```python
from build123d import *

# Parameters (mm, degrees)
SKETCH1_R           = 3.2639
BOSS_EXTRUDE1_DEPTH = 4.7752


with BuildPart() as part:
    # Sketch1 → Boss-Extrude1 (new body)
    with BuildSketch(Plane.XY):
        with BuildLine():
            Line((-76.2, 0), (0, 0))
            Line((0, 0), (0, 76.2))
            Line((0, 76.2), (-24.638, 76.2))
            Line((-24.638, 76.2), (-24.638, 27.0256))
            ThreePointArc((-24.638, 27.0256), (-25.337311849, 25.337311849), (-27.0256, 24.638))
            Line((-27.0256, 24.638), (-76.2, 24.638))
            Line((-76.2, 24.638), (-76.2, 0))
        make_face()
        with Locations((-12.7, 38.1)):
            Circle(SKETCH1_R, mode=Mode.SUBTRACT)
        with Locations((-12.7, 63.5)):
            Circle(SKETCH1_R, mode=Mode.SUBTRACT)
        with Locations((-12.7, 12.7)):
            Circle(SKETCH1_R, mode=Mode.SUBTRACT)
        with Locations((-38.1, 12.7)):
            Circle(SKETCH1_R, mode=Mode.SUBTRACT)
        with Locations((-63.5, 12.7)):
            Circle(SKETCH1_R, mode=Mode.SUBTRACT)
    extrude(amount=BOSS_EXTRUDE1_DEPTH)


solid = part.part
```
Design review of the part built by this model. Coordinates are the model's own, in mm. A direction names the side the tool comes from. Coordinates: 2 decimals unless noted, no trailing zeros. Write each loop counter-clockwise with the first axis right and the second up, starting at its lowest first coordinate (ties: lowest second). Pieces come first, ordered by that corner, then holes. Notation, with made-up numbers: M 64,13 L 97,13 A29 ccw 97,41 Z; hole C 35,40.25 d2. An arc over 180 degrees is marked long. Answer as a JSON object with one key per item and string values.
Item 1: Draft analysis for pull direction X (two halves, no side actions). For faces 1 (the flat face through (-30, 22, 4.775)), 2 (the cylindrical face through (-13.125, 41.336, 2.354)), 3 (the cylindrical face through (-25.319, 25.356, 2.354)), state which applies: pulls with the +X half, pulls with the -X half, needs draft (parallel to the pull), parting line crosses it, or undercut.
Outcome:
{"face 1": "needs draft", "face 2": "undercut", "face 3": "pulls with the -X half"}
Item 2: Add section C-C, the plane z = 3.95. Give the boundary of the cut face in (x, y), and give its area (3 significant figures).
Outcome:
{"outline": "M -76.2,0 L 0,0 L 0,76.2 L -24.64,76.2 L -24.64,27.03 A2.39 cw -27.03,24.64 L -76.2,24.64 Z; hole C -63.5,12.7 d6.53; hole C -38.1,12.7 d6.53; hole C -12.7,12.7 d6.53; hole C -12.7,38.1 d6.53; hole C -12.7,63.5 d6.53", "area": "2,980 mm²"}
Item 3: Add section A-A, the plane y = 12.7. Give the boundary of the cut face in (x, z), and give its area (3 significant figures).
Outcome:
{"outline": "M -76.2,0 L -66.76,0 L -66.76,4.78 L -76.2,4.78 Z; M -60.24,0 L -41.36,0 L -41.36,4.78 L -60.24,4.78 Z; M -34.84,0 L -15.96,0 L -15.96,4.78 L -34.84,4.78 Z; M -9.44,0 L 0,0 L 0,4.78 L -9.44,4.78 Z", "area": "270 mm²"}
Item 4: Add section D-D, the plane x = -38.1. Give the boundary of the cut face in (y, z).
Outcome:
{"outline": "M 0,0 L 9.44,0 L 9.44,4.78 L 0,4.78 Z; M 15.96,0 L 24.64,0 L 24.64,4.78 L 15.96,4.78 Z"}
Item 5: Machinability: for faces 4 (the flat face through (-39, 0, 2)), 5 (the flat face through (-51, 24.638, 2)), which of the approach directions +Z, -Z, +X, -X, +Y, -Y give a long, thin tool a straight path to every point of the face, cutting with its end or side? Answer none if there is none.
Outcome:
{"face 4": "+Z, -Z, +X, -X, -Y", "face 5": "+Z, -Z, -X, +Y"}
Item 6: Wall thickness on probe 1 along Y at (x, z) = (-12.7, 3.3); probe 2 along Y at (x, z) = (-63.5, 3.85); probe 3 along Y at (x, z) = (-49, 3.75): over which ranges is each line inside the solid? List them lowest first.
Outcome:
{"probe 1": "0 to 9.44, 15.96 to 34.84, 41.36 to 60.24, 66.76 to 76.2", "probe 2": "0 to 9.44, 15.96 to 24.64", "probe 3": "0 to 24.64"}
Item 7: Insertion check: pin 1 Ø1.4 at (x, z) = (-53, 2.5) entering from +Y. The pin has a flat end and moves straight along its axis. Give the tip position at first contact, or say it passes through.
Outcome:
{"pin 1": "y = 24.64"}
Item 8: Add section B-B, the plane y = 63.5. Give the boundary of the cut face in (x, z).
Outcome:
{"outline": "M -24.64,0 L -15.96,0 L -15.96,4.78 L -24.64,4.78 Z; M -9.44,0 L 0,0 L 0,4.78 L -9.44,4.78 Z"}
